Source: CAD feature listing. Evaluate the final solid. Frame: model axes, mm. Face numbers are marked on the shaded views. A direction names the side the tool comes from. Coordinates: 2 decimals unless noted, no trailing zeros. Write each loop counter-clockwise with the first axis right and the second up, starting at its lowest first coordinate (ties: lowest second). Pieces come first, ordered by that corner, then holes. Notation, with made-up numbers: (57, -11) -> (86, -11) arc R17 cw to (86, 9) -> close; hole circle Ø10 at (35.5, -28). An arc over 180 degrees is marked (long way). One line per item, written item: value. Start each with the question number.
1. Section query D-D, the plane z = -4. Output: boundary loops of the cut face in (x, y), and give its area (3 significant figures).
2. Section query C-C, the plane y = 70.5. Output: boundary loops of the cut face in (x, z), and give its area (3 significant figures).
3. Section query A-A, the plane x = -2.5. Output: boundary loops of the cut face in (y, z).
4. First-contact query: P1, Ø5, axis at x = -7.5, y = 56, coming from the +Z side; P2, Ø9, axis at y = 71.5, z = 0.5, coming from the +X side; P3, Ø4, axis at x = -2.5, z = -9, coming from the +Y side. Flat tips, straight axial feed; report the tip coordinate or a pass-through.
5. Mould query, pull axis Y, two halves, no side actions, for the marked faces 1, 2 and 3. Classes: released by +Y, released by -Y, zero draft, split by the parting line, or undercut.
6. Access query for the marked faces 4, 5, 6 and 7. Directions: +Z, -Z, +X, -X, +Y, -Y. A direction counts if a zero-diameter tool reaches every point of the face in a straight line with its end or side. Return the directions, or none.
7. Section query B-B, the plane x = 6.5. Output: boundary loops of the cut face in (y, z), and give its area (3 significant figures).
8. Line query: line 1 (Y direction, x = -8, z = 0); line 2 (Y direction, x = 6.5, z = 1); line 3 (Y direction, x = 39.5, z = -4.25). Output: solid intervals per line, ascending.
from build123d import *

# Parameters (mm, degrees)
CROQUIS1_R              = 2
SALIENTE_EXTRUIR1_DEPTH = 12.7
CROQUIS2_W              = 10.3
CROQUIS2_H              = 11
SALIENTE_EXTRUIR2_DEPTH = 8.5
CROQUIS3_R              = 3
CORTAR_EXTRUIR1_DEPTH   = 9.5


with BuildPart() as part:
    # Croquis1 → Saliente-Extruir1 (new body, symmetric)
    with BuildSketch(Plane.XY):
        Polygon((13, 65), (43, 65), (43, 0), (0, 0), (0, 65), (0, 76), (13, 76), align=None)
        with Locations((39.5, 4)):
            Circle(CROQUIS1_R, mode=Mode.SUBTRACT)
        with Locations((6.5, 70.5)):
            Circle(CROQUIS1_R, mode=Mode.SUBTRACT)
    extrude(amount=SALIENTE_EXTRUIR1_DEPTH, both=True)

    # Croquis2 → Saliente-Extruir2 (add, symmetric)
    with BuildSketch(Plane.XY):
        with Locations((-5.15, 58.5)):
            Rectangle(CROQUIS2_W, CROQUIS2_H)
        with Locations((-5.15, 17.5)):
            Rectangle(CROQUIS2_W, CROQUIS2_H)
    extrude(amount=SALIENTE_EXTRUIR2_DEPTH, both=True)

    # Croquis3 → Cortar-Extruir1 (cut)
    with BuildSketch(Plane.ZY.offset(10.3)):
        with Locations((0, 58.5)):
            Circle(CROQUIS3_R)
        with Locations((0, 17.5)):
            Circle(CROQUIS3_R)
    extrude(amount=-CORTAR_EXTRUIR1_DEPTH, mode=Mode.SUBTRACT)


solid = part.part
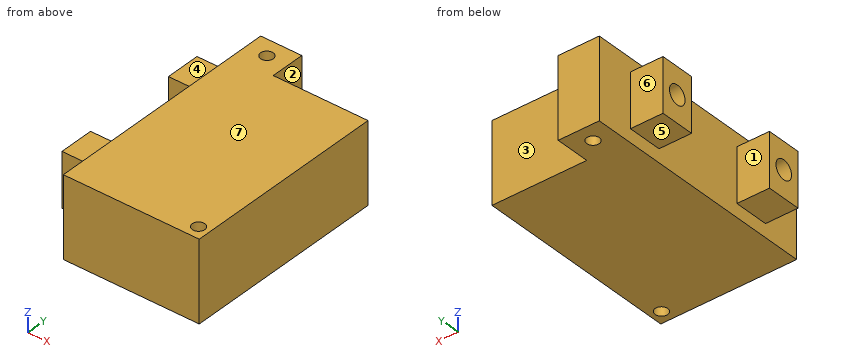
Computed values:
1. outline: (-10.3, 12) -> (0, 12) -> (0, 0) -> (43, 0) -> (43, 65) -> (13, 65) -> (13, 76) -> (0, 76) -> (0, 64) -> (-10.3, 64) -> (-10.3, 53) -> (0, 53) -> (0, 23) -> (-10.3, 23) -> close; hole circle Ø4 at (6.5, 70.5); hole circle Ø4 at (39.5, 4)
1. area: 3,140 mm²
2. outline: (0, -12.7) -> (4.5, -12.7) -> (4.5, 12.7) -> (0, 12.7) -> close; (8.5, -12.7) -> (13, -12.7) -> (13, 12.7) -> (8.5, 12.7) -> close
2. area: 229 mm²
3. outline: (12, -8.5) -> (23, -8.5) -> (23, 8.5) -> (12, 8.5) -> close; (53, -8.5) -> (64, -8.5) -> (64, 8.5) -> (53, 8.5) -> close; hole circle Ø6 at (17.5, 0); hole circle Ø6 at (58.5, 0)
4. P1: stops at z = 8.5
4. P2: stops at x = 13
4. P3: stops at y = 64
5. face 1: undercut
5. face 2: zero draft
5. face 3: released by +Y
6. face 4: +Z, -X, +Y, -Y
6. face 5: -Z, -X, +Y, -Y
6. face 6: +Z, -Z, -X, +Y
6. face 7: +Z, +X, -X, +Y, -Y
7. outline: (0, -12.7) -> (68.5, -12.7) -> (68.5, 12.7) -> (0, 12.7) -> close; (72.5, -12.7) -> (76, -12.7) -> (76, 12.7) -> (72.5, 12.7) -> close
7. area: 1,830 mm²
8. line 1: y = 12 to 14.5, 20.5 to 23, 53 to 55.5, 61.5 to 64
8. line 2: y = 0 to 68.5, 72.5 to 76
8. line 3: y = 0 to 2, 6 to 65
